Model file for the job. Use its own axes, mm. A direction names the side the tool comes from. Round coordinates to 2 decimals unless told otherwise and drop trailing zeros. Loops run counter-clockwise (first coordinate to the right, second up) from the corner with the lowest first, then second, coordinate; pieces in that order, holes last. Notation, with made-up numbers: (14, 82) - (39, 82) arc R9 cw to (39, 96) - close; hole circle Ø11 at (72.25, 86.5). An arc over 180 degrees is marked (long way). Answer as a JSON object with one key per item and string values.
from build123d import *

# Parameters (mm, degrees)
F0_W         = 35
F0_H         = 27
F1_DEPTH     = 15
F2_DEPTH     = 2
F3_T1_DEPTH  = 20
F3_T3_DEPTH  = 31
F3_T5_DEPTH  = 23
F3_S9_W      = 2
F3_S9_H      = 2
F3_T10_DEPTH = 2
F3_S15_W     = 2
F3_S15_H     = 2
F3_T16_DEPTH = 2
F3_S21_W     = 2
F3_S21_H     = 2
F3_T22_DEPTH = 2
F3_S27_W     = 2
F3_S27_H     = 2
F3_T28_DEPTH = 2


# Not quite as in the source:
# - a fillet or chamfer that OpenCascade refuses, or shapes differently, is made with other operations: its cross-section is extruded or revolved along the edge and cut away or added


with BuildPart() as f1:
    # F0 (on Top) → F1 (new body)
    with BuildSketch(Plane.XY):
        with Locations((-13.2022674233, 7.6325895488)):
            Rectangle(F0_W, F0_H)
        with BuildLine():
            Line((-14.73041686, 19.4694728107), (-0.7022674233, 17.1325895488))
            Line((-0.7022674233, 17.1325895488), (-0.7022674233, 7.6325895488))
            Line((-0.7022674233, 7.6325895488), (-0.7022674233, -1.8674104512))
            Line((-0.7022674233, -1.8674104512), (-14.73041686, -4.2042937131))
            ThreePointArc((-14.73041686, -4.2042937131), (-24.4591286842, -1.5233431387), (-28.7022674233, 7.6325895488))
            ThreePointArc((-28.7022674233, 7.6325895488), (-24.4591286842, 16.7885222364), (-14.73041686, 19.4694728107))
        make_face(mode=Mode.SUBTRACT)
    extrude(amount=F1_DEPTH)

    # F0 (on Top) → F2 (join)
    with BuildSketch(Plane.XY):
        with Locations((-13.2022674233, 7.6325895488)):
            Rectangle(F0_W, F0_H)
        with BuildLine():
            Line((-14.73041686, 19.4694728107), (-0.7022674233, 17.1325895488))
            Line((-0.7022674233, 17.1325895488), (-0.7022674233, 7.6325895488))
            Line((-0.7022674233, 7.6325895488), (-0.7022674233, -1.8674104512))
            Line((-0.7022674233, -1.8674104512), (-14.73041686, -4.2042937131))
            ThreePointArc((-14.73041686, -4.2042937131), (-24.4591286842, -1.5233431387), (-28.7022674233, 7.6325895488))
            ThreePointArc((-28.7022674233, 7.6325895488), (-24.4591286842, 16.7885222364), (-14.73041686, 19.4694728107))
        make_face(mode=Mode.SUBTRACT)
        with BuildLine():
            ThreePointArc((-14.73041686, -4.2042937131), (-7.5463347357, -0.1242717121), (-4.7022674233, 7.6325895488))
            Line((-4.7022674233, 7.6325895488), (-28.7022674233, 7.6325895488))
            ThreePointArc((-28.7022674233, 7.6325895488), (-24.4591286842, -1.5233431387), (-14.73041686, -4.2042937131))
        make_face()
        with BuildLine():
            ThreePointArc((-4.7022674233, 7.6325895488), (-7.5463347357, 15.3894508097), (-14.73041686, 19.4694728107))
            ThreePointArc((-14.73041686, 19.4694728107), (-24.4591286842, 16.7885222364), (-28.7022674233, 7.6325895488))
            Line((-28.7022674233, 7.6325895488), (-4.7022674233, 7.6325895488))
        make_face()
        with BuildLine():
            Line((-0.7022674233, 7.6325895488), (-0.7022674233, 17.1325895488))
            Line((-0.7022674233, 17.1325895488), (-14.73041686, 19.4694728107))
            ThreePointArc((-14.73041686, 19.4694728107), (-7.5463347357, 15.3894508097), (-4.7022674233, 7.6325895488))
            Line((-4.7022674233, 7.6325895488), (-0.7022674233, 7.6325895488))
        make_face()
        with BuildLine():
            Line((-0.7022674233, -1.8674104512), (-0.7022674233, 7.6325895488))
            Line((-0.7022674233, 7.6325895488), (-4.7022674233, 7.6325895488))
            ThreePointArc((-4.7022674233, 7.6325895488), (-7.5463347357, -0.1242717121), (-14.73041686, -4.2042937131))
            Line((-14.73041686, -4.2042937131), (-0.7022674233, -1.8674104512))
        make_face()
    extrude(amount=-F2_DEPTH)

    # F3: fillet of radius 2 on 8 edges, made by hand

    # F3_s2 → F3_t1 (cut)
    with BuildSketch(Plane.XY.offset(-7)):
        with BuildLine():
            ThreePointArc((-30.7022674233, -3.8674104512), (-30.1164809856, -5.2816240135), (-28.7022674233, -5.8674104512))
            Line((-28.7022674233, -5.8674104512), (-30.7022674233, -5.8674104512))
            Line((-30.7022674233, -5.8674104512), (-30.7022674233, -3.8674104512))
        make_face()
        with BuildLine():
            ThreePointArc((4.2977325767, -3.8674104512), (3.7119461391, -5.2816240135), (2.2977325767, -5.8674104512))
            Line((2.2977325767, -5.8674104512), (4.2977325767, -5.8674104512))
            Line((4.2977325767, -5.8674104512), (4.2977325767, -3.8674104512))
        make_face()
        with BuildLine():
            ThreePointArc((4.2977325767, 19.1325895488), (3.7119461391, 20.5468031112), (2.2977325767, 21.1325895488))
            Line((2.2977325767, 21.1325895488), (4.2977325767, 21.1325895488))
            Line((4.2977325767, 21.1325895488), (4.2977325767, 19.1325895488))
        make_face()
        with BuildLine():
            ThreePointArc((-30.7022674233, 19.1325895488), (-30.1164809856, 20.5468031112), (-28.7022674233, 21.1325895488))
            Line((-28.7022674233, 21.1325895488), (-30.7022674233, 21.1325895488))
            Line((-30.7022674233, 21.1325895488), (-30.7022674233, 19.1325895488))
        make_face()
    extrude(amount=F3_T1_DEPTH, mode=Mode.SUBTRACT)

    # F3_s4 → F3_t3 (cut)
    with BuildSketch(Plane.YZ.offset(-28.7022674233)):
        with BuildLine():
            ThreePointArc((-3.8674104512, 15), (-5.2816240135, 14.4142135624), (-5.8674104512, 13))
            Line((-5.8674104512, 13), (-5.8674104512, 15))
            Line((-5.8674104512, 15), (-3.8674104512, 15))
        make_face()
        with BuildLine():
            ThreePointArc((21.1325895488, 13), (20.5468031112, 14.4142135624), (19.1325895488, 15))
            Line((19.1325895488, 15), (21.1325895488, 15))
            Line((21.1325895488, 15), (21.1325895488, 13))
        make_face()
    extrude(amount=F3_T3_DEPTH, mode=Mode.SUBTRACT)

    # F3_s6 → F3_t5 (cut)
    with BuildSketch(Plane.XZ.offset(-19.1325895488)):
        with BuildLine():
            ThreePointArc((4.2977325767, 13), (3.7119461391, 14.4142135624), (2.2977325767, 15))
            Line((2.2977325767, 15), (4.2977325767, 15))
            Line((4.2977325767, 15), (4.2977325767, 13))
        make_face()
        with BuildLine():
            ThreePointArc((-30.7022674233, 13), (-30.1164809856, 14.4142135624), (-28.7022674233, 15))
            Line((-28.7022674233, 15), (-30.7022674233, 15))
            Line((-30.7022674233, 15), (-30.7022674233, 13))
        make_face()
    extrude(amount=F3_T5_DEPTH, mode=Mode.SUBTRACT)


with BuildPart() as f3_tool8:
    # F3_s9 → F3_t10 (new body)
    with BuildSketch(Plane.YZ.offset(-28.7022674233)):
        with Locations((-4.8674104512, 14)):
            Rectangle(F3_S9_W, F3_S9_H)
    extrude(amount=-F3_T10_DEPTH)

    # F3_s11 → F3_t12 (revolve, cut)
    with BuildSketch(Plane(origin=(-28.7022674233, -3.8674104512, 13), x_dir=(0, 0.7071067812, -0.7071067812), z_dir=(0, 0.7071067812, 0.7071067812))):
        with BuildLine():
            ThreePointArc((0, -2), (2, 0), (0, 2))
            Line((0, 2), (0, -2))
        make_face()
    revolve(axis=Axis((-28.7022674233, -3.8674104512, 13), (-1, 0, 0)), mode=Mode.SUBTRACT)


with BuildPart() as f1_1:
    add(f1.part)

    # F3_t7: cut F3_tool8
    add(f3_tool8.part, mode=Mode.SUBTRACT)


with BuildPart() as f3_tool14:
    # F3_s15 → F3_t16 (new body)
    with BuildSketch(Plane.YZ.offset(2.2977325767)):
        with Locations((-4.8674104512, 14)):
            Rectangle(F3_S15_W, F3_S15_H)
    extrude(amount=F3_T16_DEPTH)

    # F3_s17 → F3_t18 (revolve, cut)
    with BuildSketch(Plane(origin=(2.2977325767, -3.8674104512, 13), x_dir=(0, 0.7071067812, -0.7071067812), z_dir=(0, -0.7071067812, -0.7071067812))):
        with BuildLine():
            ThreePointArc((0, -2), (2, 0), (0, 2))
            Line((0, 2), (0, -2))
        make_face()
    revolve(axis=Axis((2.2977325767, -3.8674104512, 13), (1, 0, 0)), mode=Mode.SUBTRACT)


with BuildPart() as f1_2:
    add(f1_1.part)

    # F3_t13: cut F3_tool14
    add(f3_tool14.part, mode=Mode.SUBTRACT)


with BuildPart() as f3_tool20:
    # F3_s21 → F3_t22 (new body)
    with BuildSketch(Plane.YZ.offset(2.2977325767)):
        with Locations((20.1325895488, 14)):
            Rectangle(F3_S21_W, F3_S21_H)
    extrude(amount=F3_T22_DEPTH)

    # F3_s23 → F3_t24 (revolve, cut)
    with BuildSketch(Plane(origin=(2.2977325767, 19.1325895488, 13), x_dir=(0, -0.7071067812, -0.7071067812), z_dir=(0, -0.7071067812, 0.7071067812))):
        with BuildLine():
            ThreePointArc((0, -2), (2, 0), (0, 2))
            Line((0, 2), (0, -2))
        make_face()
    revolve(axis=Axis((2.2977325767, 19.1325895488, 13), (1, 0, 0)), mode=Mode.SUBTRACT)


with BuildPart() as f1_3:
    add(f1_2.part)

    # F3_t19: cut F3_tool20
    add(f3_tool20.part, mode=Mode.SUBTRACT)


with BuildPart() as f3_tool26:
    # F3_s27 → F3_t28 (new body)
    with BuildSketch(Plane.YZ.offset(-28.7022674233)):
        with Locations((20.1325895488, 14)):
            Rectangle(F3_S27_W, F3_S27_H)
    extrude(amount=-F3_T28_DEPTH)

    # F3_s29 → F3_t30 (revolve, cut)
    with BuildSketch(Plane(origin=(-28.7022674233, 19.1325895488, 13), x_dir=(0, -0.7071067812, -0.7071067812), z_dir=(0, 0.7071067812, -0.7071067812))):
        with BuildLine():
            ThreePointArc((0, -2), (2, 0), (0, 2))
            Line((0, 2), (0, -2))
        make_face()
    revolve(axis=Axis((-28.7022674233, 19.1325895488, 13), (-1, 0, 0)), mode=Mode.SUBTRACT)


with BuildPart() as f1_4:
    add(f1_3.part)

    # F3_t25: cut F3_tool26
    add(f3_tool26.part, mode=Mode.SUBTRACT)


solid = f1_4.part
1) Slice it at D-D on x = -18.5. List the corners of the cut face in (y, z), then the cut area to 3 significant figures.
Values follow:
{"outline": "(-5.87, -2) - (21.13, -2) - (21.13, 13) arc R2 ccw to (19.5, 14.97) - (19.5, 0) - (-4.23, 0) - (-4.23, 14.97) arc R2 ccw to (-5.87, 13) - close", "area": "101 mm²"}
2) Drop a flat-ended pin along its axis: P1, Ø7, axis at x = -19, y = 13, coming from the +Z side. Give the stop position or say it passes through.
Values follow:
{"P1": "z = 0"}
3) Probe probe 1 along X at (y, z) = (2.5, 9.25); probe 2 along Z at (x, y) = (-18, 7); probe 3 along Y at (x, z) = (-23.5, 9.25). List the from-to ranges inside material, lowest first.
Values follow:
{"probe 1": "-30.7 to -27.55, -0.7 to 4.3", "probe 2": "-2 to 0", "probe 3": "-5.87 to -2.26, 17.52 to 21.13"}
4) Two-plate mould, pull along Y, no slides. Class faces 1 (the flat face through (-26, -1, 15)), 2 (the cylindrical face through (3.727, -5.266, 5.395)), 3 (the flat face through (-7.815, 18.317, 7.395)): pulls with the +Y half, pulls with the -Y half, needs draft (parallel to the pull), parting line crosses it, or undercut.
Values follow:
{"face 1": "needs draft", "face 2": "pulls with the -Y half", "face 3": "undercut"}
5) Slice it at C-C on y = 11.25. List the corners of the cut face in (x, z).
Values follow:
{"outline": "(-30.7, -2) - (4.3, -2) - (4.3, 13) arc R2 ccw to (2.3, 15) - (-0.7, 15) - (-0.7, 0) - (-28.14, 0) - (-28.14, 15) - (-28.7, 15) arc R2 ccw to (-30.7, 13) - close"}
6) Slice it at A-A on z = 0.75. List the corners of the cut face in (x, y), then the cut area to 3 significant figures.
Values follow:
{"outline": "(-30.7, -3.87) arc R2 ccw to (-28.7, -5.87) - (2.3, -5.87) arc R2 ccw to (4.3, -3.87) - (4.3, 19.13) arc R2 ccw to (2.3, 21.13) - (-28.7, 21.13) arc R2 ccw to (-30.7, 19.13) - close; hole (-14.73, -4.2) - (-0.7, -1.87) - (-0.7, 17.13) - (-14.73, 19.47) arc R12 ccw (long way) to start", "area": "369 mm²"}
7) Slice it at B-B on x = -26. List the corners of the cut face in (y, z).
Values follow:
{"outline": "(-5.87, -2) - (21.13, -2) - (21.13, 13) arc R2 ccw to (19.13, 15) - (15.22, 15) - (15.22, 0) - (0.05, 0) - (0.05, 15) - (-3.87, 15) arc R2 ccw to (-5.87, 13) - close"}
8) Tool access for faces 4 (the flat face through (-30.702, 7, 6)), 5 (the flat face through (-0.702, 8, 7)): list every direction of +Z, -Z, +X, -X, +Y, -Y with a clear straight run to the whole face (end or side of a thin tool).
Values follow:
{"face 4": "+Z, -Z, -X, +Y, -Y", "face 5": "+Z"}
